Geometry check sheet. Reference: the model listing, model coordinates, mm. A direction names the side the tool comes from. Coordinates: 2 decimals unless noted, no trailing zeros. Loops run counter-clockwise (first coordinate to the right, second up) from the corner with the lowest first, then second, coordinate; pieces in that order, holes last.
from build123d import *

# Parameters (mm, degrees)
F0_W     = 15
F0_H     = 5
F1_DEPTH = 110
F2_W     = 8
F2_H     = 98.8297045976
F2_W_2   = 37
F2_H_2   = 91.1702954024
F2_W_3   = 10
F3_DEPTH = 100


# Not quite as in the source:
# - a feature of the source that left no trace in its solid (it failed there, or was rolled back) is left out


with BuildPart() as f1:
    # F0 (on Right) → F1 (new body)
    with BuildSketch(Plane.YZ):
        Polygon((30.635715595, 45.1382968587), (0, 27.4507582131), (0, 15.9037528294), (36.4732290688, 36.9615814504), align=None)
        Polygon((56.5512701892, 60.1006492799), (30.635715595, 45.1382968587), (36.4732290688, 36.9615814504), (61.5512701892, 51.4403952421), align=None)
        Polygon((15.1663048896, 66.8065926908), (0, 58.0503224802), (0, 46.5033170964), (21.0038183633, 58.6298772825), align=None)
        Polygon((43.3012701892, 83.0503224802), (15.1663048896, 66.8065926908), (21.0038183633, 58.6298772825), (48.3012701892, 74.3900684424), align=None)
        Polygon((-20, -101.9496775198), (-20, -96.9496775198), (-20, -81.9496775198), (-25, -81.9496775198), (-25, -101.9496775198), align=None)
        with Locations((-12.5, -99.4496775198)):
            Rectangle(F0_W, F0_H)
        Polygon((0, 88.0503224802), (-5, 88.0503224802), (-5, -96.9496775198), (-5, -101.9496775198), (0, -101.9496775198), (0, -10), (0, 0), (0, 15.9037528294), (0, 27.4507582131), (0, 46.5033170964), (0, 58.0503224802), align=None)
        Polygon((0, 0), (0, -10), (70, -10), (62.860808794, 0), align=None)
    extrude(amount=F1_DEPTH)

    # F2 (on Front) → F3 (cut)
    with BuildSketch(Plane.XZ):
        with Locations((51, 64.6969747171)):
            Rectangle(F2_W, F2_H)
        with Locations((59, 64.6969747171)):
            Rectangle(F2_W, F2_H)
        with Locations((91.5, -30.3030252829)):
            Rectangle(F2_W_2, F2_H_2)
        with Locations((18.5, -30.3030252829)):
            Rectangle(F2_W_2, F2_H_2)
        with Locations((42, -30.3030252829)):
            Rectangle(F2_W_3, F2_H_2)
        with Locations((68, -30.3030252829)):
            Rectangle(F2_W_3, F2_H_2)
        with Locations((91.5, 64.6969747171)):
            Rectangle(F2_W_2, F2_H)
        with Locations((18.5, 64.6969747171)):
            Rectangle(F2_W_2, F2_H)
    extrude(amount=-F3_DEPTH, mode=Mode.SUBTRACT)


solid = f1.part
1) Access from +Z, -Z, +X, -X, +Y, -Y to the whole of each face (thin tool, end or side, straight path). Record for faces 1 (the flat face through (55, 35, -10)), 2 (the flat face through (54, -13, -96.95)), 3 (the flat face through (63, 22, 66)), 4 (the flat face through (37, 31, 38)), 5 (the flat face through (47, 35, -5)).
Data:
face 1: -Z, +X, -X, +Y
face 2: +Z, +X, -X
face 3: +Z, +Y
face 4: +Z, -Z, -X, +Y
face 5: -Z, -X, +Y
2) Mould release check, pull along Y, two halves, no side actions. Record for faces 6 (the flat face through (67.93, 28.671, 44.004)), 7 (the flat face through (41.93, 45.836, 78.66)), 8 (the flat face through (54, -13, -101.95)): +Y half, -Y half, draft (parallel to the pull), parting line (faces both ways), or undercut.
Data:
face 6: undercut
face 7: +Y half
face 8: draft
3) Section check A-A on x = 8.5. Record the cut outline in (y, z).
Data:
outline: (-25, -101.95) - (0, -101.95) - (0, 88.05) - (-5, 88.05) - (-5, -96.95) - (-20, -96.95) - (-20, -81.95) - (-25, -81.95) - close
4) Material ranges on probe 1 along X at (y, z) = (28, 66); probe 2 along Y at (x, z) = (56, -46.5); probe 3 along Z at (x, y) = (77.5, -15), recorded low to high.
Data:
probe 1: x = 37 to 47, 63 to 73
probe 2: y = -5 to 0
probe 3: z = -101.95 to -96.95
5) Section check C-C on z = -4.5. Record the cut outline in (x, y).
Data:
outline: (0, -5) - (110, -5) - (110, 0) - (63, 0) - (63, 66.07) - (47, 66.07) - (47, 0) - (0, 0) - close
6) Depth check by flat-ended pin: pin 1 (5 mm diameter, centred on x = 52, z = -35, fed in from -Y); pin 2 (10 mm diameter, centred on y = -3.5, z = 11.5, fed in from -X); pin 3 (2.5 mm diameter, centred on x = 42, y = -21.5, fed in from +Z); pin 4 (22 mm diameter, centred on y = 28, z = 47, fed in from +X). Enter the tip coordinate at first touch or a pass-through.
Data:
pin 1: stops at y = -5
pin 2: stops at x = 0
pin 3: stops at z = -81.95
pin 4: stops at x = 73
7) Section check B-B on y = 54.5. Record the cut outline in (x, z), and give its area (3 significant figures).
Data:
outline: (37, 47.37) - (47, 47.37) - (47, 58.92) - (37, 58.92) - close; (47, -10) - (63, -10) - (63, 0) - (47, 0) - close; (63, 47.37) - (73, 47.37) - (73, 58.92) - (63, 58.92) - close
area: 391 mm2
8) Section check D-D on y = 10. Record the cut outline in (x, z), and give its area (3 significant figures).
Data:
outline: (37, 21.68) - (47, 21.68) - (47, 33.22) - (37, 33.22) - close; (37, 52.28) - (47, 52.28) - (47, 63.82) - (37, 63.82) - close; (47, -10) - (63, -10) - (63, 0) - (47, 0) - close; (63, 21.68) - (73, 21.68) - (73, 33.22) - (63, 33.22) - close; (63, 52.28) - (73, 52.28) - (73, 63.82) - (63, 63.82) - close
area: 622 mm2
